CAD build for the part. Positions are in the model's coordinates, mm. Face numbers are marked on the shaded views. A direction names the side the tool comes from. Give positions to 0.01 mm unless a question says otherwise; leave off trailing zeros. Write each loop counter-clockwise with the first axis right and the second up, starting at its lowest first coordinate (ties: lowest second). Pieces come first, ordered by that corner, then holes. Notation, with made-up numbers: (-7, -2) - (36, -2) arc R15 ccw to (36, 25) - close; hole circle Ø2 at (-38, 79). An arc over 180 degrees is marked (long way). Answer as a JSON object with one key per item and string values.
from build123d import *

# Parameters (mm, degrees)
F0_W     = 215
F0_H     = 34.0627696488
F0_W_2   = 207.1483027775
F0_H_2   = 31.7993836311
F3_DEPTH = 336
F4_SIZE  = 5
F5_SIZE  = 5
F7_DEPTH = 30
F8_SIZE  = 2


with BuildPart() as f1:
    # F0 (on Front) → F1 (revolve)
    with BuildSketch(Plane.XZ):
        Polygon((-91.5524632784, 42.0493356358), (41.045925168, 42.0493356358), (41.045925168, 171.5008825727), (41.045925168, 367.6874935627), (-133.954074832, 367.6874935627), (-133.954074832, 42.0493356358), align=None)
        Polygon((-173.954074832, 0), (41.045925168, 0), (41.045925168, 42.0493356358), (-91.5524632784, 42.0493356358), align=None)
        with Locations((-66.454074832, -17.0313848244)):
            Rectangle(F0_W, F0_H)
        Polygon((-173.954074832, -89.0246674962), (-166.1023776095, -89.0246674962), (41.045925168, -89.0246674962), (41.045925168, -34.0627696488), (-173.954074832, -34.0627696488), align=None)
        with Locations((-62.5282262207, -104.9243593118)):
            Rectangle(F0_W_2, F0_H_2)
    revolve(axis=Axis((41.045925168, 0, -11.5101449135), (0, 0, -1)))

    # F2 (on face) → F3 (join)
    with BuildSketch(Plane.XY.offset(367.6874935627)):
        with BuildLine():
            Line((41.045925296, 175), (-133.954074832, 175))
            Line((-133.954074832, 175), (-133.954074832, -4.69e-07))
            ThreePointArc((-133.954074832, -4.69e-07), (-82.6977616602, 123.7436865871), (41.045925296, 175))
        make_face()
        with BuildLine():
            ThreePointArc((216.045925168, 0), (164.7896119209, 123.7436866624), (41.045925296, 175))
            ThreePointArc((41.045925296, 175), (-82.6977616602, 123.7436865871), (-133.954074832, -4.69e-07))
            ThreePointArc((-133.954074832, -4.69e-07), (-82.6977616199, -123.7436866274), (41.0459244719, -175))
            ThreePointArc((41.0459244719, -175), (164.7896116296, -123.7436869538), (216.045925168, 0))
        make_face()
        with BuildLine():
            Line((216.045925168, 175), (41.045925296, 175))
            ThreePointArc((41.045925296, 175), (164.7896119209, 123.7436866624), (216.045925168, 0))
            Line((216.045925168, 0), (216.045925168, 175))
        make_face()
        with BuildLine():
            Line((216.045925168, -175), (216.045925168, 0))
            ThreePointArc((216.045925168, 0), (164.7896116296, -123.7436869538), (41.0459244719, -175))
            Line((41.0459244719, -175), (216.045925168, -175))
        make_face()
        with BuildLine():
            ThreePointArc((41.0459244719, -175), (-82.6977616199, -123.7436866274), (-133.954074832, -4.69e-07))
            Line((-133.954074832, -4.69e-07), (-133.954074832, -175))
            Line((-133.954074832, -175), (41.0459244719, -175))
        make_face()
    extrude(amount=-F3_DEPTH)

    # F4
    f4_edges = [f1.edges().sort_by_distance(p)[0] for p in [
        (41.045925, 175, 31.687494),
        (-133.954075, 0, 31.687494),
        (216.045925, 0, 31.687494),
        (41.045925, -175, 31.687494),
    ]]
    chamfer(f4_edges, length=F4_SIZE)

    # F5
    f5_edges = [f1.edges().sort_by_distance(p)[0] for p in [
        (216.045925, 175, 202.187494),
        (216.045925, -175, 202.187494),
        (-133.954075, 175, 202.187494),
        (-133.954075, -175, 202.187494),
    ]]
    chamfer(f5_edges, length=F5_SIZE)

    # F6 (on face) → F7 (join)
    with BuildSketch(Plane.XZ.offset(175)):
        Polygon((-33.954074832, 367.6874935627), (-33.954074832, 36.6874935627), (116.045925168, 36.6874935627), (116.045925168, 367.6874935627), (41.0459247854, 367.6874935627), align=None)
    extrude(amount=F7_DEPTH)

    # F8
    f8_edges = [f1.edges().sort_by_distance(p)[0] for p in [
        (-33.954075, -205, 202.187494),
        (116.045925, -205, 202.187494),
    ]]
    chamfer(f8_edges, length=F8_SIZE)


solid = f1.part
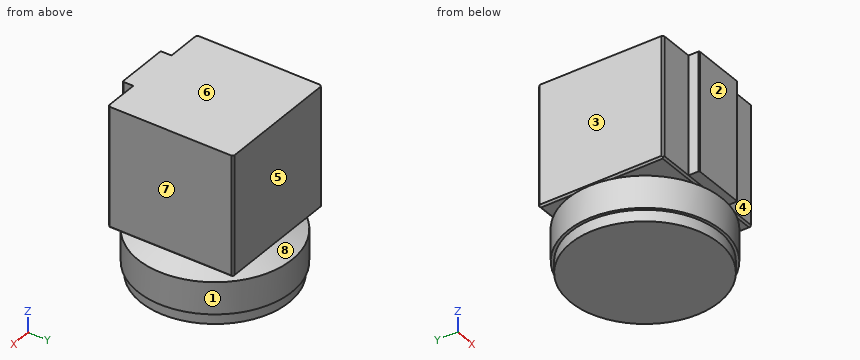
Item 1: Cut at B-B (y = 0). Give the cut face in (x, z), and give its area (3 significant figures).
Entries:
{"outline": "(-173.95, -89.02) - (-166.1, -89.02) - (-166.1, -120.82) - (248.19, -120.82) - (248.19, -89.02) - (256.05, -89.02) - (256.05, 0) - (193.95, 31.69) - (211.05, 31.69) - (216.05, 36.69) - (216.05, 367.69) - (-133.95, 367.69) - (-133.95, 36.69) - (-128.95, 31.69) - (-111.86, 31.69) - (-173.95, 0) - close", "area": "181,000 mm2"}
Item 2: Flat gauge pins, fed straight in: P1, Ø12, axis at x = 58.5, z = -21, coming from the +Y side; P2, Ø1, axis at y = -142.5, z = 192, coming from the -X side; P3, Ø6, axis at y = -98, z = 110.5, coming from the +X side. Where does each tip first touch, or does it go through?
Entries:
{"P1": "y = 214.69", "P2": "x = -133.95", "P3": "x = 216.05"}
Item 3: Cut at C-C (z = -33). Give the cut face in (x, y).
Entries:
{"outline": "circle Ø430 at (41.05, 0)"}
Item 4: Which spindle directions (+Z, -Z, +X, -X, +Y, -Y) get a long thin tool onto all of the face, cutting with end or side? Do the marked faces 1, 2, 3, 4 and 5. Say none if no direction does.
Entries:
{"face 1": "-Z", "face 2": "+Z, +X, -X, -Y", "face 3": "+Z, -X, +Y, -Y", "face 4": "+Z, +X, -Y", "face 5": "+Z, +X, -X, +Y"}
Item 5: Mould opens along Z. For the marked faces 6, 7 and 8 say: +Z half, -Z half, draft (parallel to the pull), parting line (faces both ways), or undercut.
Entries:
{"face 6": "+Z half", "face 7": "draft", "face 8": "undercut"}
Item 6: Probe line 1 (Y direction, x = 27, z = 295); line 2 (Y direction, x = -107, z = 87.5); line 3 (X direction, y = -40, z = 78). List the from-to ranges inside material, lowest first. Write a range as from..to.
Entries:
{"line 1": "-205..175", "line 2": "-175..175", "line 3": "-133.95..216.05"}
Item 7: Cut at A-A (z = 147.5). Give the cut face in (x, y), and give its area (3 significant figures).
Entries:
{"outline": "(-133.95, -170) - (-128.95, -175) - (-33.95, -175) - (-33.95, -203) - (-31.95, -205) - (114.05, -205) - (116.05, -203) - (116.05, -175) - (211.05, -175) - (216.05, -170) - (216.05, 170) - (211.05, 175) - (-128.95, 175) - (-133.95, 170) - close", "area": "127,000 mm2"}
